Check sheet for the modelled part. Datum: model origin and axes. Units: mm. A direction names the side the tool comes from. Give positions to 0.01 mm unless a question says otherwise; leave off trailing zeros. Write each loop counter-clockwise with the first axis right and the second up, starting at its lowest first coordinate (ties: lowest second). Pieces come first, ordered by that corner, then holes.
from build123d import *

# Parameters (mm, degrees)
SKETCH1_W                        = 685.8
SKETCH1_H                        = 22.225
BASE_FLANGE1_DEPTH               = 2.65684
EDGE_FLANGE1_DEPTH               = 685.8
EDGE_FLANGE2_DEPTH               = 685.8
F_17_64_0_26563_DIAMETER_HOLE1_D = 6.747002
F_10_0_1935_DIAMETER_HOLE1_D     = 4.9149
F_10_0_1935_DIAMETER_HOLE1_DEPTH = 2.65684
FILLET1_R                        = 2.54


# Sheet-metal steps are written as plain solids
with BuildPart() as part:
    # Sketch1 → Base-Flange1 (new body)
    with BuildSketch(Plane(origin=(0, 0, 0), x_dir=(1, 0, 0), z_dir=(0, 1, 0))):
        with Locations((342.9, 11.1125)):
            Rectangle(SKETCH1_W, SKETCH1_H)
    extrude(amount=-BASE_FLANGE1_DEPTH)

    # Edge-Flange1 section (across the edge) → Edge-Flange1 (add)
    with BuildSketch(Plane(origin=(0, 0, 3.175), x_dir=(0, 0, -1), z_dir=(1, 0, 0))):
        with BuildLine():
            Line((-2.65684, 3.175), (-2.65684, 41.79316))
            Line((-2.65684, 41.79316), (0, 41.79316))
            Line((0, 41.79316), (0, 3.175))
            ThreePointArc((0, 3.175), (0.92993597, 0.92993597), (3.175, 0))
            Line((3.175, 0), (3.175, -2.65684))
            ThreePointArc((3.175, -2.65684), (-0.948733611, -0.948733611), (-2.65684, 3.175))
        make_face()
    extrude(amount=EDGE_FLANGE1_DEPTH)

    # Edge-Flange2 section (across the edge) → Edge-Flange2 (add)
    with BuildSketch(Plane(origin=(685.8, 0, -25.4), x_dir=(0, 0, 1), z_dir=(-1, 0, 0))):
        with BuildLine():
            Line((-2.65684, 3.175), (-2.65684, 41.79316))
            Line((-2.65684, 41.79316), (0, 41.79316))
            Line((0, 41.79316), (0, 3.175))
            ThreePointArc((0, 3.175), (0.92993597, 0.92993597), (3.175, 0))
            Line((3.175, 0), (3.175, -2.65684))
            ThreePointArc((3.175, -2.65684), (-0.948733611, -0.948733611), (-2.65684, 3.175))
        make_face()
    extrude(amount=EDGE_FLANGE2_DEPTH)

    # 17/64 (0.26563) Diameter Hole1 (through all)
    with Locations(Plane(origin=(0, 0, -28.05684), x_dir=(-1, 0, 0), z_dir=(0, 0, -1))):
        with Locations((-342.9, 22.74316)):
            Hole(F_17_64_0_26563_DIAMETER_HOLE1_D / 2)

    # #10 (0.1935) Diameter Hole1
    with Locations(Plane.XY.offset(5.83184)):
        with Locations((596.9, 13.21816), (596.9, 32.26816), (628.65, 32.26816), (628.65, 13.21816), (660.4, 13.21816), (660.4, 32.26816), (88.9, 13.21816), (88.9, 32.26816), (57.15, 13.21816), (57.15, 32.26816), (25.4, 13.21816), (25.4, 32.26816)):
            Hole(F_10_0_1935_DIAMETER_HOLE1_D / 2, depth=F_10_0_1935_DIAMETER_HOLE1_DEPTH)

    # Fillet1
    fillet1_edges = [part.edges().sort_by_distance(p)[0] for p in [
        (0, 41.79316, 4.50342),
        (685.8, 41.79316, 4.50342),
        (685.8, 41.79316, -26.72842),
        (0, 41.79316, -26.72842),
    ]]
    fillet(fillet1_edges, radius=FILLET1_R)


solid = part.part
1) Gauge pin test, flat ends, axial feed: pin 1 (4 mm diameter, centred on x = 25.4, y = 32.27, fed in from +Z); pin 2 (1.5 mm diameter, centred on y = 29, z = -23.5, fed in from -X); pin 3 (10 mm diameter, centred on x = 389.5, z = -8.5, fed in from +Y). Record the tip position at first contact, or that the pin passes through.
2) Scan lines: L1, parallel to Z at x = 353.5, y = 35 (3 decimals); L2, parallel to Y at x = 596.9, z = 4; L3, parallel to Y at x = 134, z = -10. Record each from-to range of solid material in increasing order.
3) Sectioned sample at B-B on z = -16. Record the boundary of the cut face in (x, y), then the cut area to 3 significant figures.
4) Draft check along Z on faces 3 (the flat face through (338, 22, 5.832)), 4 (the flat face through (338, -2.657, -11)), 5 (the flat face through (348, 23, -25.4)). Enter one of: +Z half, -Z half, draft (parallel to the pull), parting line (faces both ways), or undercut.
5) Access from +Z, -Z, +X, -X, +Y, -Y to the whole of each face (thin tool, end or side, straight path). Record for faces 1 (the flat face through (338, 23, 3.175)), 2 (the flat face through (685.8, -0.2, -11)).
6) Sectioned sample at A-A on x = 609. Record the boundary of the cut face in (y, z) (3 decimals), then the cut area to 3 significant figures.
Answers below:
1. pin 1: stops at z = -25.4
1. pin 2: passes through
1. pin 3: stops at y = 0
2. L1: z = -28.057 to -25.4, 3.175 to 5.832
2. L2: y = -1.07 to 10.76, 15.68 to 29.81, 34.73 to 41.79
2. L3: y = -2.66 to 0
3. outline: (0, -2.66) - (685.8, -2.66) - (685.8, 0) - (0, 0) - close
3. area: 1,820 mm2
4. face 3: +Z half
4. face 4: draft
4. face 5: undercut
5. face 1: +X, -X, +Y
5. face 2: +Z, -Z, +X, +Y, -Y
6. outline: (-2.657, -22.225) arc R5.832 ccw to (3.175, -28.057) - (41.793, -28.057) - (41.793, -25.4) - (3.175, -25.4) arc R3.175 cw to (0, -22.225) - (0, 0) arc R3.175 cw to (3.175, 3.175) - (41.793, 3.175) - (41.793, 5.832) - (3.175, 5.832) arc R5.832 ccw to (-2.657, 0) - close
6. area: 302 mm2
